```python
from build123d import *

# Parameters (mm, degrees)
SKETCH7_W                = 76.2
SKETCH7_H                = 88.9
BOSS_EXTRUDE1_DEPTH      = 57.15
BOSS_EXTRUDE2_DEPTH      = 0.127
BOSS_EXTRUDE2_DEPTH_BACK = 35.687
SKETCH8_R                = 22.352
SKETCH10_W               = 30.208401757
SKETCH10_H               = 50.8
SKETCH10_W_2             = 14.705109565
CUT_EXTRUDE2_DEPTH       = 846.764631146
SKETCH11_W               = 76.2
SKETCH11_H               = 6.35
BOSS_EXTRUDE3_DEPTH      = 22.86
SKETCH14_W               = 76.2
SKETCH14_H               = 6.35
BOSS_EXTRUDE4_DEPTH      = 63.5
SKETCH12_R               = 3.2766
CUT_EXTRUDE3_DEPTH       = 720.944943326
RIB5_REACH               = 897.713
SKETCH17_WALL_W          = 1900.017933472
SKETCH17_WALL_H          = 3.81


with BuildPart() as part:
    # Sketch7 → Boss-Extrude1 (new body)
    with BuildSketch(Plane(origin=(0, 474.726, 0), x_dir=(1, 0, 0), z_dir=(0, 1, 0))):
        with Locations((0, -608.711)):
            Rectangle(SKETCH7_W, SKETCH7_H)
    extrude(amount=BOSS_EXTRUDE1_DEPTH)


with BuildPart() as body_2:
    # Sketch8 → Boss-Extrude2 (new, two sides: drawn at the far end of the back side and taken through both)
    with BuildSketch(Plane(origin=(0, -83.644613765, 474.372177356), x_dir=(-1, 0, 0), z_dir=(2.9130205458871294e-15, 0.17364817766694987, -0.9848077530122047)).offset(-BOSS_EXTRUDE2_DEPTH_BACK)):
        with Locations(Location((0, 634.503351151, 0), (0, 0, 90))):
            Circle(SKETCH8_R)
    extrude(amount=BOSS_EXTRUDE2_DEPTH + BOSS_EXTRUDE2_DEPTH_BACK)


with BuildPart() as part_1:
    add(part.part)

    # Combine1: cut body 2
    add(body_2.part, mode=Mode.SUBTRACT)

    # Sketch10 → Cut-Extrude2 (cut, through all)
    with BuildSketch(Plane(origin=(38.1, 0, 0), x_dir=(0, 0, -1), z_dir=(1, 0, 0))):
        with Locations((-638.056799122, 506.476)):
            Rectangle(SKETCH10_W, SKETCH10_H)
        with Locations((-571.613554783, 506.476)):
            Rectangle(SKETCH10_W_2, SKETCH10_H)
    extrude(amount=-CUT_EXTRUDE2_DEPTH, mode=Mode.SUBTRACT)

    # Sketch11 → Boss-Extrude3 (add)
    with BuildSketch(Plane(origin=(0, 0, 564.261), x_dir=(-1, 0, 0), z_dir=(0, 0, -1))):
        with Locations((0, 477.901)):
            Rectangle(SKETCH11_W, SKETCH11_H)
    extrude(amount=BOSS_EXTRUDE3_DEPTH)

    # Sketch14 → Boss-Extrude4 (add)
    with BuildSketch(Plane.XY.offset(653.161)):
        with Locations((0, 477.901)):
            Rectangle(SKETCH14_W, SKETCH14_H)
    extrude(amount=BOSS_EXTRUDE4_DEPTH)

    # Sketch12 → Cut-Extrude3 (cut, through all)
    with BuildSketch(Plane.XZ.offset(-474.726)):
        with Locations((0, 703.961)):
            Circle(SKETCH12_R)
        with Locations((0, 551.561)):
            Circle(SKETCH12_R)
    extrude(amount=-CUT_EXTRUDE3_DEPTH, mode=Mode.SUBTRACT)

    # Sketch17 wall → Rib5 (add, up to next)
    with BuildSketch(Plane(origin=(38.1, 506.476, 669.806799122), x_dir=(0, 0.476582557871, -0.879129720538), z_dir=(0, 0.879129720538, 0.476582557871)), mode=Mode.PRIVATE) as rib5_sk1:
        with Locations((0, 1.905)):
            Rectangle(SKETCH17_WALL_W, SKETCH17_WALL_H)
    rib5_tool1 = extrude(rib5_sk1.sketch, amount=-RIB5_REACH, mode=Mode.PRIVATE) - part_1.part
    rib5 = rib5_tool1.solids().sort_by_distance((38.1, 506.476, 669.806799122))[0]
    add(rib5)

    # Mirror1: Rib5 across plane
    add(rib5.mirror(Plane(origin=(0, 0, 0), x_dir=(0, 0, 1), z_dir=(1, 0, 0))))


solid = part_1.part
```
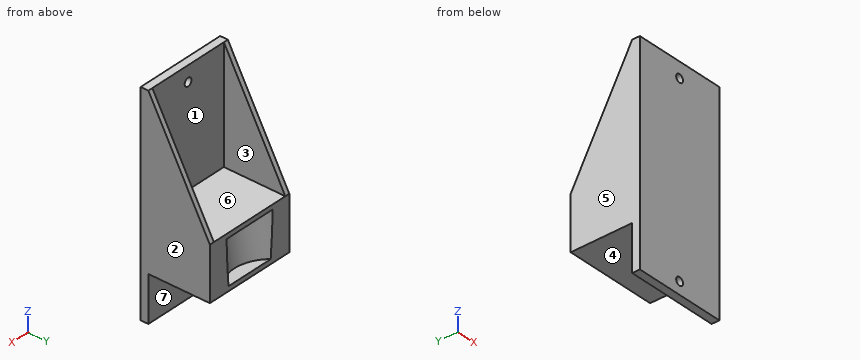
CAD build for the part. Positions are in the model's coordinates, mm. Face numbers are marked on the shaded views. A direction names the side the tool comes from. Give positions to 0.01 mm unless a question says otherwise; leave off trailing zeros. Loops run counter-clockwise (first coordinate to the right, second up) from the corner with the lowest first, then second, coordinate; pieces in that order, holes last. Notation, with made-up numbers: M 73,49.5 L 117,49.5 A12 cw 117,59.5 Z; hole C -32,-23 d8. An arc over 180 degrees is marked long. Use one line per item in the form item = value.
Item 1: Two-plate mould, pull along X, no slides. Class the marked faces 1, 2, 3 and 4: pulls with the +X half, pulls with the -X half, needs draft (parallel to the pull), parting line crosses it, or undercut.
Determined:
face_1 = undercut
face_2 = pulls with the +X half
face_3 = undercut
face_4 = needs draft
Item 2: Flat gauge pins, fed straight in: pin 1 (4 mm diameter, centred on x = 11.5, z = 691, fed in from +Y); pin 2 (8 mm diameter, centred on y = 497.5, z = 576, fed in from +X); pin 3 (5 mm diameter, centred on x = 0, z = 551.561, fed in from -Y); pin 4 (2 mm diameter, centred on x = -11, y = 525, fed in from -Z). Where does each tip first touch, or does it go through?
Determined:
pin_1 = 481.08
pin_2 = 38.1
pin_3 = through
pin_4 = 578.97
Item 3: Slice it at C-C (x = 31). List the corners of the cut face in (y, z), plus the area to 3 significant figures.
Determined:
outline = M 474.73,541.4 L 481.08,541.4 L 481.08,578.97 L 531.88,578.97 L 531.88,622.95 L 481.08,622.95 L 481.08,716.66 L 474.73,716.66 Z
area = 3,350 mm2
Item 4: Drill centre lines: probe 1 along Z at (x, y) = (0, 478); probe 2 along X at (y, z) = (481.5, 688.5); probe 3 along Z at (x, y) = (-16, 509.5). Where is each one in solid material? Low to high. Write a range as from..to.
Determined:
probe_1 = 541.4..548.28, 554.84..700.68, 707.24..716.66
probe_2 = -38.1..-34.29, 34.29..38.1
probe_3 = 578.97..622.95
Item 5: Slice it at D-D (x = 17). List the corners of the cut face in (y, z), plus the area to 3 significant figures.
Determined:
outline = M 474.73,541.4 L 481.08,541.4 L 481.08,578.97 L 531.88,578.97 L 531.88,582.78 L 526.95,581.91 L 520.73,617.18 L 531.88,619.14 L 531.88,622.95 L 481.08,622.95 L 481.08,716.66 L 474.73,716.66 Z
area = 3,060 mm2
Item 6: Slice it at A-A (x = 0). List the corners of the cut face in (y, z).
Determined:
outline = M 474.73,541.4 L 481.08,541.4 L 481.08,548.28 L 474.73,548.28 Z; M 474.73,554.84 L 481.08,554.84 L 481.08,578.97 L 531.88,578.97 L 531.88,582.78 L 519.23,580.55 L 513.01,615.82 L 531.88,619.14 L 531.88,622.95 L 481.08,622.95 L 481.08,700.68 L 474.73,700.68 Z; M 474.73,707.24 L 481.08,707.24 L 481.08,716.66 L 474.73,716.66 Z
Item 7: Which spindle directions (+Z, -Z, +X, -X, +Y, -Y) get a long thin tool onto all of the face, cutting with end or side? Do the marked faces 5, 6 and 7. Say none if no direction does.
Determined:
face_5 = +Z, -Z, -X, +Y, -Y
face_6 = +Z, +Y
face_7 = -Z, +X, -X, +Y
Item 8: Slice it at B-B (z = 658). List the corners of the cut face in (x, y).
Determined:
outline = M -38.1,474.73 L 38.1,474.73 L 38.1,512.88 L 34.29,512.88 L 34.29,481.08 L -34.29,481.08 L -34.29,512.88 L -38.1,512.88 Z
